from build123d import *

# Parameters (mm, degrees)
F1_DEPTH = 6.35
F2_R     = 1.27


with BuildPart() as f1:
    # F0 (on Top) → F1 (new body)
    with BuildSketch(Plane.XY):
        Polygon((-22.479, -11.43), (22.479, -11.43), (22.479, 11.43), (1.016, 11.43), (1.016, 6.985), (18.669, 6.985), (18.669, -6.985), (-18.669, -6.985), (-18.669, 6.985), (-1.016, 6.985), (-1.016, 11.43), (-22.479, 11.43), align=None)
        with BuildLine():
            ThreePointArc((-1.016, 6.985), (-0.302004, 9.2075), (-1.016, 11.43))
            Line((-1.016, 11.43), (-1.016, 6.985))
        make_face()
        with BuildLine():
            Line((1.016, 6.985), (1.016, 11.43))
            ThreePointArc((1.016, 11.43), (0.300607, 9.2075), (1.016, 6.985))
        make_face()
    extrude(amount=F1_DEPTH)

    # F2
    f2_edges = [f1.edges().sort_by_distance(p)[0] for p in [
        (-9.8425, 6.985, 6.35),
        (9.8425, 6.985, 6.35),
        (18.669, 0, 6.35),
        (0, -6.985, 6.35),
        (-18.669, 0, 6.35),
        (0, -6.985, 0),
        (18.669, 0, 0),
        (9.8425, 6.985, 0),
        (-9.8425, 6.985, 0),
        (-18.669, 0, 0),
        (11.7475, 11.43, 6.35),
        (-11.7475, 11.43, 6.35),
        (-22.479, 0, 6.35),
        (0, -11.43, 6.35),
        (22.479, 0, 6.35),
        (22.479, 0, 0),
        (0, -11.43, 0),
        (11.7475, 11.43, 0),
        (-11.7475, 11.43, 0),
        (-22.479, 0, 0),
    ]]
    fillet(f2_edges, radius=F2_R)


solid = f1.part
Here's how the part is built. I have some questions about the finished solid (model axes, mm). A direction names the side the tool comes from. Coordinates: 2 decimals unless noted, no trailing zeros. Write each loop counter-clockwise with the first axis right and the second up, starting at its lowest first coordinate (ties: lowest second). Pieces come first, ordered by that corner, then holes.
Item 1: If I drill on line 1 (Y direction, x = -13, z = 2) (3 decimals); line 2 (X direction, y = -6.5, z = 5); line 3 (X direction, y = 0.75, z = 5.75), over which ranges is the centre line in solid material (lowest first)?
Item 2: On a 3-axis mill with a long thin cutter (end or side, diameter ignored), from which of +Z, -Z, +X, -X, +Y, -Y can I reach the whole of each face in a straight line? I mean faces 1 (the cylindrical face through (-10.04, 7.35, 0.38)), 2 (the cylindrical face through (0.315, -11.068, 5.968)), 3 (the flat face through (-10, 6.985, 3)), 4 (the flat face through (12, 11.43, 3)), 5 (the cylindrical face through (10.32, 7.35, 5.97)). Say none if no direction works.
Item 3: Will this pin go through, and if not, where does the flat tip stop? pin 1 (12 mm diameter, centred on x = 3.5, y = 5.5, fed in from -Z).
Item 4: I want a section at B-B on x = 11.5. Write out the boundary of the cut face in (y, z) (3 decimals).
Item 5: I want a section at C-C on z = 3.25. Write out the boundary of the cut face in (x, y) (1 decimal), and give its area (3 significant figures).
Item 6: If we mould it in two halves opening along Y, with no side actions, what happens to faces 6 (the flat face through (0, -11.43, 3)), 7 (the cylindrical face through (19.031, -0.116, 0.382)), 8 (the flat face through (0, -6.985, 3)), 9 (the cylindrical face through (-11.605, 11.068, 0.382))? For each: +Y half, -Y half, draft (parallel to the pull), parting line (faces both ways), or undercut.
Item 7: I want a section at D-D on y = 7.75. Write out the boundary of the cut face in (x, z).
Item 8: I want a section at A-A on y = 5. Write out the boundary of the cut face in (x, z).
Findings below:
1. line 1: y = -11.43 to -6.985, 6.985 to 11.43
1. line 2: x = -22.48 to -18.67, 18.67 to 22.48
1. line 3: x = -22.29 to -18.86, 18.86 to 22.29
2. face 1: -Z
2. face 2: +Z, +X, -X, -Y
2. face 3: +Z, -Z
2. face 4: +Z, -Z, +X, -X, +Y
2. face 5: +Z
3. pin 1: stops at z = 0
4. outline: (-11.43, 1.27) arc R1.27 ccw to (-10.16, 0) - (-8.255, 0) arc R1.27 ccw to (-6.985, 1.27) - (-6.985, 5.08) arc R1.27 ccw to (-8.255, 6.35) - (-10.16, 6.35) arc R1.27 ccw to (-11.43, 5.08) - close; (6.985, 1.27) arc R1.27 ccw to (8.255, 0) - (10.16, 0) arc R1.27 ccw to (11.43, 1.27) - (11.43, 5.08) arc R1.27 ccw to (10.16, 6.35) - (8.255, 6.35) arc R1.27 ccw to (6.985, 5.08) - close
5. outline: (-22.5, -11.4) - (22.5, -11.4) - (22.5, 11.4) - (1, 11.4) arc R3.8 ccw to (1, 7) - (18.7, 7) - (18.7, -7) - (-18.7, -7) - (-18.7, 7) - (-1, 7) arc R3.8 ccw to (-1, 11.4) - (-22.5, 11.4) - close
5. area: 501 mm2
6. face 6: -Y half
6. face 7: undercut
6. face 8: undercut
6. face 9: +Y half
7. outline: (-22.48, 1.27) arc R1.27 ccw to (-21.21, 0) - (-19.94, 0) arc R1.27 ccw to (-19.43, 0.1) - (-0.59, 0.1) - (-0.59, 6.25) - (-19.43, 6.25) arc R1.27 ccw to (-19.94, 6.35) - (-21.21, 6.35) arc R1.27 ccw to (-22.48, 5.08) - close; (0.59, 0.1) - (19.43, 0.1) arc R1.27 ccw to (19.94, 0) - (21.21, 0) arc R1.27 ccw to (22.48, 1.27) - (22.48, 5.08) arc R1.27 ccw to (21.21, 6.35) - (19.94, 6.35) arc R1.27 ccw to (19.43, 6.25) - (0.59, 6.25) - close
8. outline: (-22.48, 1.27) arc R1.27 ccw to (-21.21, 0) - (-19.94, 0) arc R1.27 ccw to (-18.67, 1.27) - (-18.67, 5.08) arc R1.27 ccw to (-19.94, 6.35) - (-21.21, 6.35) arc R1.27 ccw to (-22.48, 5.08) - close; (18.67, 1.27) arc R1.27 ccw to (19.94, 0) - (21.21, 0) arc R1.27 ccw to (22.48, 1.27) - (22.48, 5.08) arc R1.27 ccw to (21.21, 6.35) - (19.94, 6.35) arc R1.27 ccw to (18.67, 5.08) - close
